Geometry check sheet. Reference: the model listing, model coordinates, mm. Face numbers are marked on the shaded views. A direction names the side the tool comes from. Round coordinates to 2 decimals unless told otherwise and drop trailing zeros. Loops run counter-clockwise (first coordinate to the right, second up) from the corner with the lowest first, then second, coordinate; pieces in that order, holes last. Notation, with made-up numbers: (5, -25.5) -> (15, -25.5) arc R22 cw to (15, 11.5) -> close; hole circle Ø3 at (20.25, -32). An arc over 180 degrees is marked (long way). Use a Markdown table: item, result. Add a question column.
Q1. Sectioned sample at A-A, the plane x = 0. Enter the section's corners in (y, z), then the cut area to 3 significant figures.
Q2. Material ranges on L1, parallel to X at y = -1, z = 0; L2, parallel to Y at x = 0, z = 17.35; L3, parallel to Z at x = 17, y = 17, recorded low to high.
Q3. Sectioned sample at D-D, the plane y = 27. Enter the section's corners in (x, z).
Q4. Release check for a two-part mould opening along Y. For the marked faces 3, 4 and 5 record: released by +Y, released by -Y, zero draft, split by the parting line, or undercut.
Q5. Set-up check for the marked faces 1 and 2: record each of +Z, -Z, +X, -X, +Y, -Y from which the full face is reachable in a straight line by a thin tool's end or side.
Q6. Sectioned sample at C-C, the plane z = 7.5. Enter the section's corners in (x, y).
Q7. Gauge pin test, flat ends, axial feed: P1, Ø6, axis at x = -12, y = 5, coming from the +Z side; P2, Ø15.5, axis at x = -6.5, y = 9, coming from the -Z side; P3, Ø5, axis at x = 7, z = 0.5, coming from the -Y side. Record the tip position at first contact, or that the pin passes through.
```python
from build123d import *

# Parameters (mm, degrees)
EXTRUDE_1_DEPTH          = 20
EXTRUDE_1_DEPTH_BACK     = 7
SKETCH_1_R               = 32.5
CUT_EXTRUDE_6_DEPTH      = 55
CUT_EXTRUDE_6_DEPTH_BACK = 81
SKETCH_2_R               = 26
EXTRUDE_4_DEPTH          = 16
EXTRUDE_4_DEPTH_BACK     = 3
SKETCH_3_R               = 26


with BuildPart() as part:
    # 草图1 → 凸台-拉伸1 (new, two sides: drawn at the far end of the back side and taken through both)
    with BuildSketch(Plane.XY.offset(-EXTRUDE_1_DEPTH_BACK)):
        Circle(SKETCH_1_R)
    extrude(amount=EXTRUDE_1_DEPTH + EXTRUDE_1_DEPTH_BACK)

    # 草图2 → 切除-拉伸6 (cut, two sides: drawn at the far end of the back side and taken through both)
    with BuildSketch(Plane.XY.offset(-CUT_EXTRUDE_6_DEPTH_BACK)):
        Circle(SKETCH_2_R)
    extrude(amount=CUT_EXTRUDE_6_DEPTH + CUT_EXTRUDE_6_DEPTH_BACK, mode=Mode.SUBTRACT)

    # 草图3 → 凸台-拉伸4 (add, two sides: drawn at the far end of the back side and taken through both)
    with BuildSketch(Plane.XY.offset(-EXTRUDE_4_DEPTH_BACK)):
        Circle(SKETCH_3_R)
    extrude(amount=EXTRUDE_4_DEPTH + EXTRUDE_4_DEPTH_BACK)


solid = part.part
```
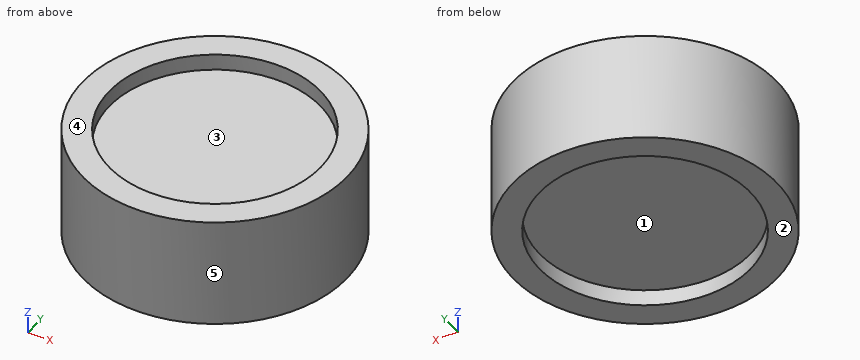
Values:
| question | item | result |
|---|---|---|
| 1 | outline | (-32.5, -7) -> (-26, -7) -> (-26, -3) -> (26, -3) -> (26, -7) -> (32.5, -7) -> (32.5, 20) -> (26, 20) -> (26, 16) -> (-26, 16) -> (-26, 20) -> (-32.5, 20) -> close |
| 1 | area | 1,340 mm^2 |
| 2 | L1 | -32.48 to 32.48 |
| 2 | L2 | -32.5 to -26, 26 to 32.5 |
| 2 | L3 | -3 to 16 |
| 3 | outline | (-18.09, -7) -> (18.09, -7) -> (18.09, 20) -> (-18.09, 20) -> close |
| 4 | face 3 | undercut |
| 4 | face 4 | zero draft |
| 4 | face 5 | split by the parting line |
| 5 | face 1 | -Z |
| 5 | face 2 | -Z, +X, -X, +Y, -Y |
| 6 | outline | circle Ø65 at (0, 0) |
| 7 | P1 | z = 16 |
| 7 | P2 | z = -3 |
| 7 | P3 | y = -32.19 |
